The model under review builds one solid part; all positions refer to its coordinate system, in mm. A direction names the side the tool comes from. Coordinates: 2 decimals unless noted, no trailing zeros. Order: outer loops, then holes, each group sorted by start corner. A loop starts at its lowest first (then second) coordinate and runs counter-clockwise, first axis right, second up. Notation, with made-up numbers: M 38.25,-0.5 L 93.25,-0.5 A32 cw 93.25,36.5 Z; hole C 48,47.5 d7. An arc over 180 degrees is marked long. Answer as CSV lines item,"result". Start each with the question number.
Q1. For P1, Ø10, axis at x = 17.5, z = 7, coming from the -Y side; P2, Ø2, axis at x = 19, z = 10, coming from the +Y side; P3, Ø2, axis at y = 10.5, z = 3, coming from the +X side; P4, Ø8, axis at y = 3.5, z = -2.5, coming from the -X side, all flat-tipped, find the tip position at first contact; note any pin that passes through.
Q2. Machinability: for faces 5 (the face through (21.235, 0.806, 10.507)), 6 (the face through (20.1, 2.5, 9.8)), 7 (the face through (4.8, 2.5, -9.8)), 8 (the face through (23.987, -0.195, -10.493)), which of the approach directions +Z, -Z, +X, -X, +Y, -Y give a long, thin tool a straight path to every point of the face, cutting with its end or side? Answer none if there is none.
Q3. Consider section A-A on y = 10. Write out the cut boundary in (x, z).
Q4. The part is to be moulded in two halves that separate along Z. For faces 1 (the face through (4, -1, -10)), 2 (the face through (24.248, -1.787, 9.493)), 3 (the face through (12.437, 11.498, 0.198)), 4 (the face through (12, 0, 9)), say which applies: +Z half, -Z half, draft (parallel to the pull), parting line (faces both ways), or undercut.
Q5. Wall thickness on L1, parallel to Z at x = 22, y = 1.5; L2, parallel to Z at x = 16.75, y = 1.5; L3, parallel to X at y = 9.5, z = -8: over which ranges is each line inside the solid? List them lowest first. Write a range as [from, to].
Q6. Consider section B-B on x = 3.25. Write out the cut boundary in (y, z), and give its area (3 significant figures).
Q7. Consider section D-D on z = -4.5. Write out the cut boundary in (x, y), and give its area (3 significant figures).
Q8. Consider section C-C on y = 3.5. Write out the cut boundary in (x, z).
from build123d import *

# Parameters (mm, degrees)
SKETCH3_W             = 2
SKETCH3_H             = 5
BOSS_EXTRUDE1_DEPTH   = 25
BOSS_EXTRUDE1_2_DEPTH = 25
SKETCH4_W             = 5
SKETCH4_H             = 5
CUT_EXTRUDE1_DEPTH    = 1
SKETCH5_W             = 5
SKETCH5_H             = 5
CUT_EXTRUDE2_DEPTH    = 1
SWEEP1_START          = 8
SWEEP1_DEPTH          = 9
SKETCH7_R             = 1.5
BOSS_EXTRUDE2_DEPTH   = 1
BOSS_EXTRUDE3_START   = 1
SKETCH8_R             = 1.5
BOSS_EXTRUDE3_DEPTH   = 1
FILLET1_R             = 2.5
CUT_EXTRUDE3_DEPTH    = 1
CUT_EXTRUDE4_DEPTH    = 1
FILLET2_R             = 2.5


# Read off the part's stored shape, not the designer's step: Sweep1
with BuildPart() as part:
    # Sketch3 → Boss-Extrude1 (new body)
    with BuildSketch(Plane(origin=(0, 0, 0), x_dir=(0, 0, -1), z_dir=(1, 0, 0))):
        with Locations((-10, 0)):
            Rectangle(SKETCH3_W, SKETCH3_H)
    extrude(amount=BOSS_EXTRUDE1_DEPTH)

    # Sketch4 → Cut-Extrude1 (cut)
    with BuildSketch(Plane.XY.offset(11)):
        with Locations((2.5, 0)):
            Rectangle(SKETCH4_W, SKETCH4_H)
        with Locations((22.5, 0)):
            Rectangle(SKETCH4_W, SKETCH4_H)
    extrude(amount=-CUT_EXTRUDE1_DEPTH, mode=Mode.SUBTRACT)



with BuildPart() as body_2:
    # Sketch3 → Boss-Extrude1 2 (new body)
    with BuildSketch(Plane(origin=(0, 0, 0), x_dir=(0, 0, -1), z_dir=(1, 0, 0))):
        with Locations((10, 0)):
            Rectangle(SKETCH3_W, SKETCH3_H)
    extrude(amount=BOSS_EXTRUDE1_2_DEPTH)

    # Sketch5 → Cut-Extrude2 (cut)
    with BuildSketch(Plane(origin=(0, 0, -11), x_dir=(-1, 0, 0), z_dir=(0, 0, -1))):
        with Locations((-22.5, 0)):
            Rectangle(SKETCH5_W, SKETCH5_H)
        with Locations((-2.5, 0)):
            Rectangle(SKETCH5_W, SKETCH5_H)
    extrude(amount=-CUT_EXTRUDE2_DEPTH, mode=Mode.SUBTRACT)


with BuildPart() as part_1:
    add(part.part)

    add(body_2.part)  # Sweep1 merges body 2
    # Sweep1 outline → Sweep1 (add)
    with BuildSketch(Plane.YZ.offset(SWEEP1_START)):
        with BuildLine():
            Line((2.5, -9), (2.5, -11))
            ThreePointArc((2.5, -11), (13.5, 0), (2.5, 11))
            Line((2.5, 11), (2.5, 9))
            ThreePointArc((2.5, 9), (11.5, 0), (2.5, -9))
        make_face()
    extrude(amount=SWEEP1_DEPTH)

    # Sketch7 → Boss-Extrude2 (add)
    with BuildSketch(Plane(origin=(0, 0, -10), x_dir=(-1, 0, 0), z_dir=(0, 0, -1))):
        with Locations(Location((-2.5, 0, 0), (0, 0, 270))):
            Circle(SKETCH7_R)
        with Locations(Location((-22.5, 0, 0), (0, 0, 90))):
            Circle(SKETCH7_R)
    extrude(amount=BOSS_EXTRUDE2_DEPTH)

    # Sketch8 → Boss-Extrude3 (add)
    with BuildSketch(Plane.XY.offset(10).offset(BOSS_EXTRUDE3_START)):
        with Locations(Location((22.5, 0, 0), (0, 0, 90))):
            Circle(SKETCH8_R)
        with Locations(Location((2.5, 0, 0), (0, 0, 270))):
            Circle(SKETCH8_R)
    extrude(amount=-BOSS_EXTRUDE3_DEPTH)

    # Fillet1
    fillet1_edges = [part_1.edges().sort_by_distance(p)[0] for p in [
        (0, -2.5, 9.5),
        (25, -2.5, 9.5),
        (25, -2.5, -9.5),
        (0, -2.5, -9.5),
    ]]
    fillet(fillet1_edges, radius=FILLET1_R)

    # Sketch9 → Cut-Extrude3 (cut)
    with BuildSketch(Plane.XY.offset(11)):
        Polygon((5, 2.5), (7.5, -2.5), (5, -2.5), align=None)
    extrude(amount=-CUT_EXTRUDE3_DEPTH, mode=Mode.SUBTRACT)

    # Sketch10 → Cut-Extrude4 (cut)
    with BuildSketch(Plane(origin=(0, 0, -11), x_dir=(-1, 0, 0), z_dir=(0, 0, -1))):
        Polygon((-5, 2.5), (-7.5, -2.5), (-5, -2.5), align=None)
    extrude(amount=-CUT_EXTRUDE4_DEPTH, mode=Mode.SUBTRACT)

    # Fillet2
    fillet2_edges = [part_1.edges().sort_by_distance(p)[0] for p in [
        (20, -2.5, 10.5),
        (20, -2.5, -10.5),
    ]]
    fillet(fillet2_edges, radius=FILLET2_R)


solid = part_1.part
Evaluation:
1,P1,"stops at y = -2.5"
1,P2,"stops at y = 2.5"
1,P3,"stops at x = 17"
1,P4,"passes through"
2,face 5,"+Z"
2,face 6,"+Z, -Z, +X, +Y"
2,face 7,"+Z, -Z, -X, +Y"
2,face 8,"-Z"
3,outline,"M 8,-8.05 L 17,-8.05 L 17,-4.97 L 8,-4.97 Z; M 8,4.97 L 17,4.97 L 17,8.05 L 8,8.05 Z"
4,face 1,"-Z half"
4,face 2,"draft"
4,face 3,"undercut"
4,face 4,"undercut"
5,L1,"z = [-10, -9], [9, 10]"
5,L2,"z = [-11, -9], [9, 11]"
5,L3,"x = [8, 17]"
6,outline,"M -2.5,-10 L -1.3,-10 L -1.3,-11 L 1.3,-11 L 1.3,-10 L 2.5,-10 L 2.5,-9 L -2.5,-9 Z; M -2.5,9 L 2.5,9 L 2.5,10 L 1.3,10 L 1.3,11 L -1.3,11 L -1.3,10 L -2.5,10 Z"
6,area,"15.2 mm²"
7,outline,"M 8,10.29 L 17,10.29 L 17,12.54 L 8,12.54 Z"
7,area,"20.2 mm²"
8,outline,"M 8,-10.95 L 17,-10.95 L 17,-8.94 L 8,-8.94 Z; M 8,8.94 L 17,8.94 L 17,10.95 L 8,10.95 Z"
